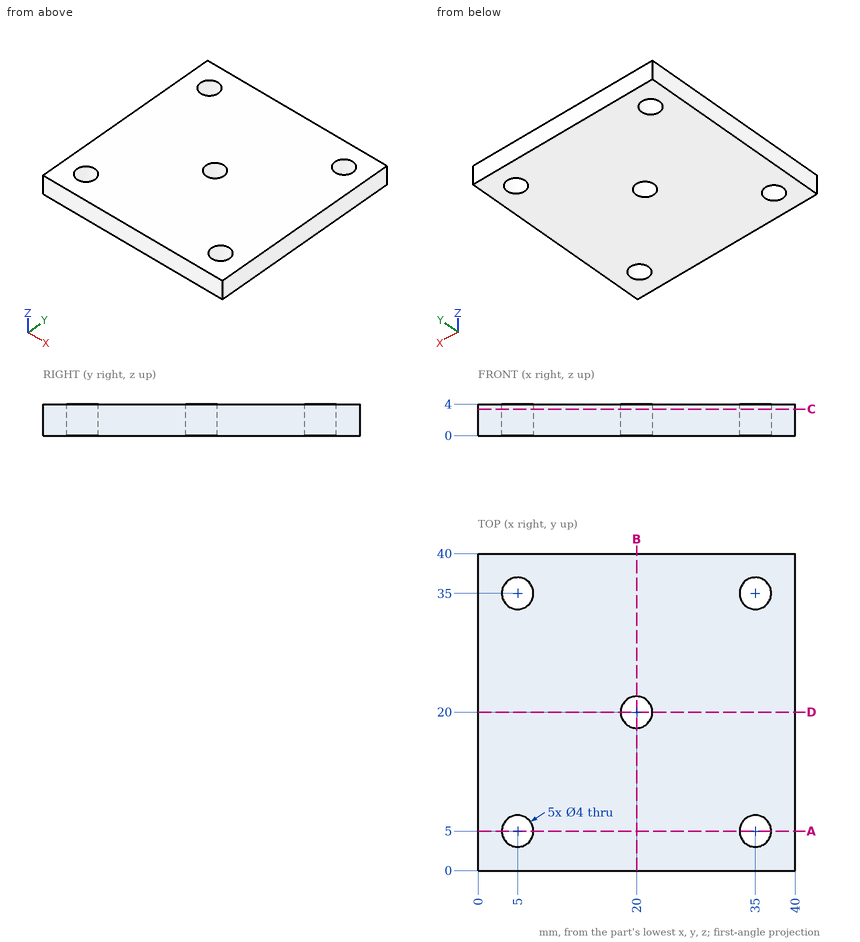
Here's the drawing with two shaded views (mm, measured from the low corner). I have some questions. Give positions to 0.01 mm unless a question says otherwise; leave off trailing zeros. Write each loop counter-clockwise with the first axis right and the second up, starting at its lowest first coordinate (ties: lowest second). Pieces come first, ordered by that corner, then holes. Notation, with made-up numbers: (10, 10) -> (34, 10) arc R26 cw to (34, 38) -> close; hole circle Ø9 at (-29.75, -24). An arc over 180 degrees is marked (long way). Use one line per item in the form item = value.
1) Suppose I cut it at A-A (y = 5). Please give me the cut outline in (x, z).
Verdict:
outline = (0, 0) -> (3, 0) -> (3, 4) -> (0, 4) -> close; (7, 0) -> (33, 0) -> (33, 4) -> (7, 4) -> close; (37, 0) -> (40, 0) -> (40, 4) -> (37, 4) -> close
2) If I drill on L1, parallel to Y at x = 35, z = 1.85; L2, parallel to Y at x = 20, z = 2.75; L3, parallel to Y at x = 34.5, z = 2, over which ranges is the centre line in solid material (lowest first)? Write a range as [from, to].
Verdict:
L1 = [0, 3], [7, 33], [37, 40]
L2 = [0, 18], [22, 40]
L3 = [0, 3.06], [6.94, 33.06], [36.94, 40]
3) Suppose I cut it at B-B (x = 20). Please give me the cut outline in (y, z), and give its area (3 significant figures).
Verdict:
outline = (0, 0) -> (18, 0) -> (18, 4) -> (0, 4) -> close; (22, 0) -> (40, 0) -> (40, 4) -> (22, 4) -> close
area = 144 mm2
4) Suppose I cut it at C-C (z = 3.35). Please give me the cut outline in (x, y), and give its area (3 significant figures).
Verdict:
outline = (0, 0) -> (40, 0) -> (40, 40) -> (0, 40) -> close; hole circle Ø4 at (5, 5); hole circle Ø4 at (5, 35); hole circle Ø4 at (20, 20); hole circle Ø4 at (35, 5); hole circle Ø4 at (35, 35)
area = 1,540 mm2
